from build123d import *

# Parameters (mm, degrees)
SKETCH1_R           = 86.995
SKETCH1_R_2         = 3.302
BOSS_EXTRUDE1_DEPTH = 2.54


with BuildPart() as part:
    # Sketch1 → Boss-Extrude1 (new body)
    with BuildSketch(Plane.YZ):
        with Locations(Location((0, 0, 0), (0, 0, 270))):
            Circle(SKETCH1_R)
        with Locations(Location((26.867048584, 71.849001137, 0), (0, 0, 270))):
            Circle(SKETCH1_R_2, mode=Mode.SUBTRACT)
        with Locations(Location((64.045308925, 34.670740796, 0), (0, 0, 270))):
            Circle(SKETCH1_R_2, mode=Mode.SUBTRACT)
        with Locations(Location((71.849001137, -26.867048584, 0), (0, 0, 270))):
            Circle(SKETCH1_R_2, mode=Mode.SUBTRACT)
        with Locations(Location((34.670740796, -64.045308925, 0), (0, 0, 270))):
            Circle(SKETCH1_R_2, mode=Mode.SUBTRACT)
        with Locations(Location((-26.867048584, -71.849001137, 0), (0, 0, 270))):
            Circle(SKETCH1_R_2, mode=Mode.SUBTRACT)
        with Locations(Location((-64.045308925, -34.670740796, 0), (0, 0, 270))):
            Circle(SKETCH1_R_2, mode=Mode.SUBTRACT)
        with Locations(Location((-71.849001137, 26.867048584, 0), (0, 0, 270))):
            Circle(SKETCH1_R_2, mode=Mode.SUBTRACT)
        with Locations(Location((-34.670740796, 64.045308925, 0), (0, 0, 270))):
            Circle(SKETCH1_R_2, mode=Mode.SUBTRACT)
    extrude(amount=BOSS_EXTRUDE1_DEPTH)


solid = part.part
Here's how the part is built. I have some questions about the finished solid (model axes, mm). Round coordinates to 2 decimals unless told otherwise and drop trailing zeros. Write each loop counter-clockwise with the first axis right and the second up, starting at its lowest first coordinate (ties: lowest second). Pieces come first, ordered by that corner, then holes.
1. Suppose I cut it at C-C (y = 48). List the corners of the cut face in (x, z) for me.
2. Suppose I cut it at A-A (z = 63.5). List the corners of the cut face in (x, y) for me, and give its area (3 significant figures).
3. If we mould it in two halves opening along Y, with no side actions, what happens to faces 1 (the cylindrical face through (1.252, -84.926, 18.859)), 2 (the cylindrical face through (1.252, 75.123, -26.437)), 3 (the flat face through (2.54, 1, 1))? For each: released by +Y, released by -Y, zero draft, split by the parting line, or undercut.
4. Suppose I cut it at D-D (z = -26). List the corners of the cut face in (x, y) for me.
5. Suppose I cut it at B-B (x = 1.8). State how many separate pieces and enclosed holes the cut face has, and give its area (3 significant figures).
6. I need wall thicknesses on L1, parallel to Z at x = 1.5, y = 0.5; L2, parallel to Z at x = 1.65, y = -53.5; L3, parallel to Z at x = 0.95, y = -66.5. Which ranges of each line are inside material? Lowest first, please.
7. Will these pins go through, and if not, where does the flat tip stop? pin 1 Ø6 at (y, z) = (64.05, 34.67) entering from +X; pin 2 Ø1.5 at (x, z) = (1.5, 20) entering from -Y.
Answer sheet:
1. outline: (0, -72.55) - (2.54, -72.55) - (2.54, 72.55) - (0, 72.55) - close
2. outline: (0, -59.46) - (2.54, -59.46) - (2.54, -37.93) - (0, -37.93) - close; (0, -31.41) - (2.54, -31.41) - (2.54, 59.46) - (0, 59.46) - close
2. area: 286 mm2
3. face 1: split by the parting line
3. face 2: undercut
3. face 3: zero draft
4. outline: (0, -83.02) - (2.54, -83.02) - (2.54, 68.66) - (0, 68.66) - close; (0, 75.04) - (2.54, 75.04) - (2.54, 83.02) - (0, 83.02) - close
5. separate pieces: 1
5. enclosed holes: 8
5. area: 23,500 mm2
6. L1: z = -86.99 to 86.99
6. L2: z = -68.6 to 68.6
6. L3: z = -56.09 to -36.88, -32.46 to 56.09
7. pin 1: passes through
7. pin 2: stops at y = -84.84
